Can you work these out from the drawing? Everything is in mm from the part's minimum corner. A direction names the side the tool comes from. Round coordinates to 2 decimals unless told otherwise and drop trailing zeros. Order: outer loops, then holes, each group sorted by start corner. A loop starts at its lowest first (then second) coordinate and runs counter-clockwise, first axis right, second up. Notation, with made-up numbers: M -22.75,38.25 L 8.25,38.25 A21 ccw 8.25,56.25 Z; hole C 13,58.25 d9. An arc over 180 degrees is marked long. Write each question's results on one line, items separated by ' | '. Start each with the question number.
1. For the marked faces 1, 2 and 3, which set-ups out of +Z, -Z, +X, -X, +Y, -Y let a thin tool reach every point of the face, with its end or its side?
2. Suppose I cut it at C-C on x = 2. Write out the boundary of the cut face in (y, z) (1 decimal).
3. Suppose I cut it at D-D on z = 1.25. Write out the boundary of the cut face in (x, y), and give its area (3 significant figures).
4. Please list where these lines run through material, in increasing order: L1, parallel to Y at x = 11.5, z = 8.25; L2, parallel to X at y = 18.75, z = 9; L3, parallel to Y at x = 4, z = 5.5.
5. Suppose I cut it at A-A on x = 29. Write out the boundary of the cut face in (y, z).
6. I'm going to push flat-ended pins straight in: pin 1 (2 mm diameter, centred on y = 14.5, z = 7, fed in from +X); pin 2 (3.5 mm diameter, centred on x = 29.79, z = 6, fed in from +Y); pin 3 (3 mm diameter, centred on x = 7, z = 9.5, fed in from +Y); pin 4 (2.5 mm diameter, centred on x = 2.21, z = 6, fed in from -Y). Where does each tip first touch, or does it pass through?
7. Suppose I cut it at B-B on y = 23.5. Write out the boundary of the cut face in (x, z), and give its area (3 significant figures).
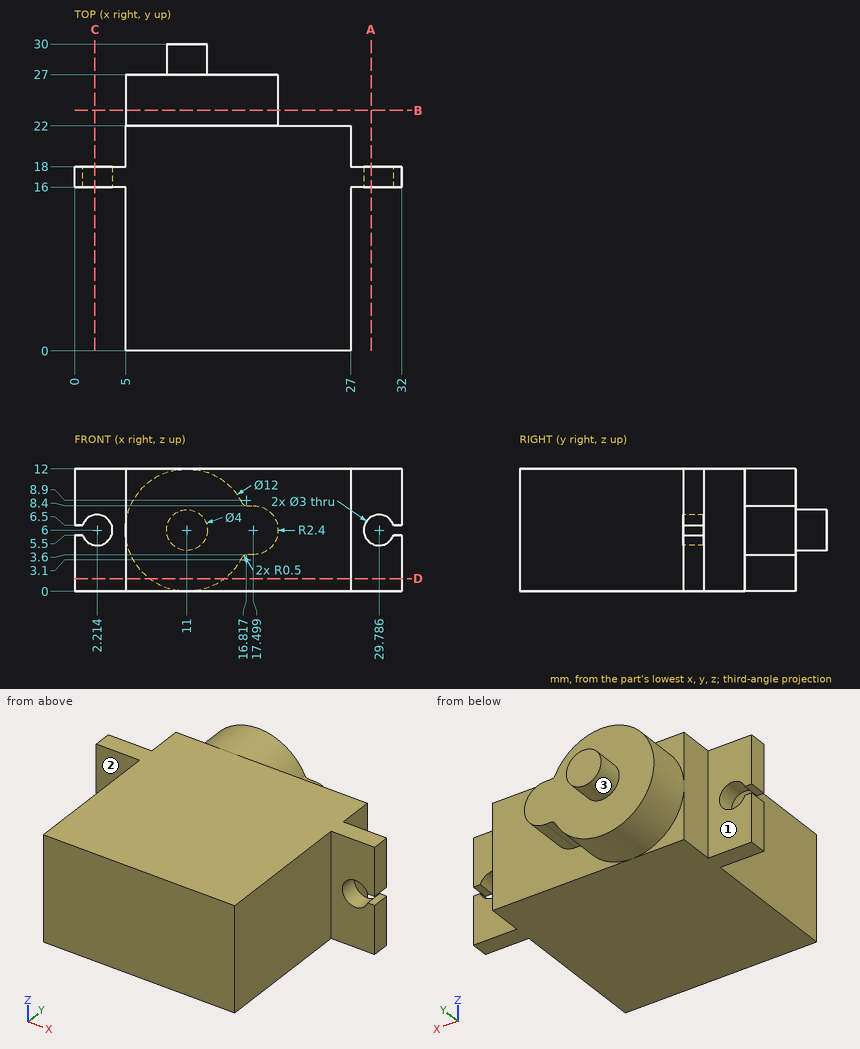
Filled sheet:
1) face 1: +Z, -Z, -X, +Y | face 2: +Z, -Z, -X, -Y | face 3: +Y
2) outline: M 16,0 L 18,0 L 18,4.5 L 16,4.5 Z; M 16,7.5 L 18,7.5 L 18,12 L 16,12 Z
3) outline: M 0,16 L 5,16 L 5,0 L 27,0 L 27,16 L 32,16 L 32,18 L 27,18 L 27,22 L 14.67,22 L 14.67,27 L 7.33,27 L 7.33,22 L 5,22 L 5,18 L 0,18 Z | area: 541 mm^2
4) L1: y = 0 to 27 | L2: x = 5 to 27 | L3: y = 16 to 18
5) outline: M 16,0 L 18,0 L 18,4.72 L 16,4.72 Z; M 16,7.28 L 18,7.28 L 18,12 L 16,12 Z
6) pin 1: stops at x = 27 | pin 2: stops at y = 18 | pin 3: stops at y = 27 | pin 4: passes through
7) outline: M 16.37,3.32 A0.5 cw 16.82,3.6 L 17.5,3.6 A2.4 ccw 17.5,8.4 L 16.82,8.4 A0.5 cw 16.37,8.68 A6 ccw long Z | area: 125 mm^2
